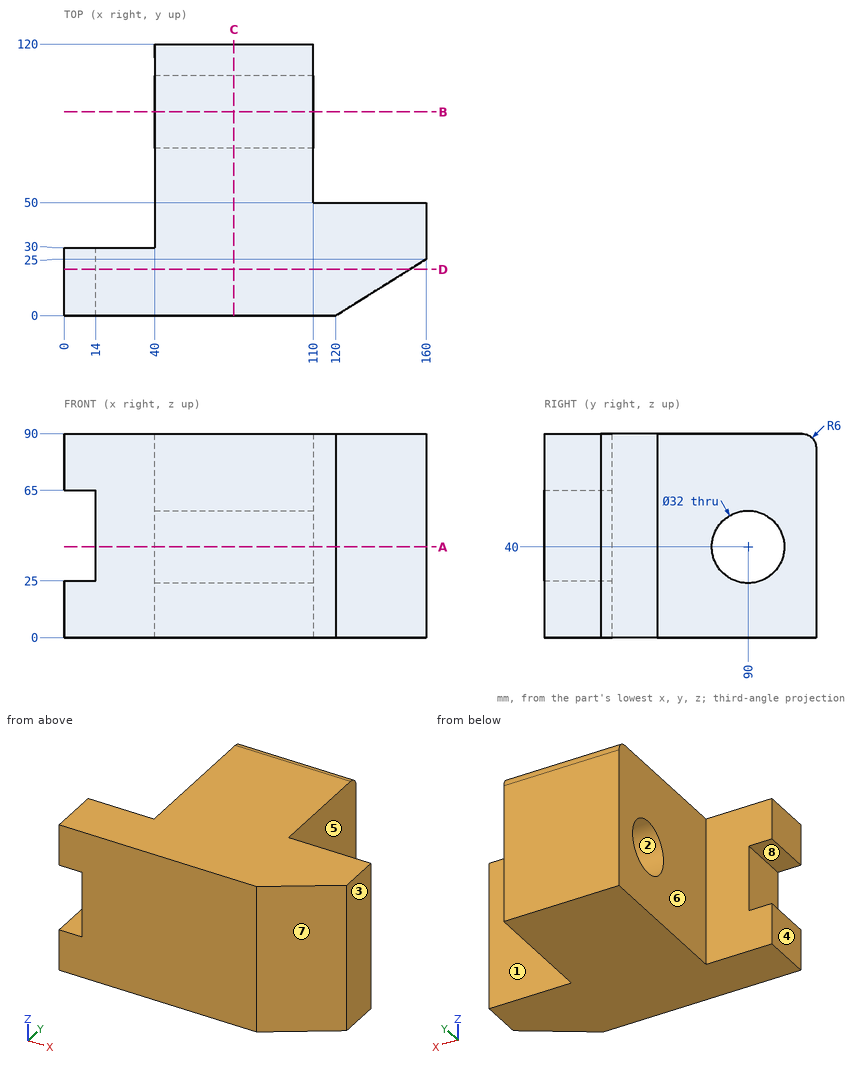
Here's the drawing with two shaded views (mm, measured from the low corner). I have some questions. A direction names the side the tool comes from. Give positions to 0.01 mm unless a question says otherwise; leave off trailing zeros. Loops run counter-clockwise (first coordinate to the right, second up) from the corner with the lowest first, then second, coordinate; pieces in that order, holes last. Notation, with made-up numbers: M 22.25,29 L 42.25,29 A25 ccw 42.25,54 Z; hole C 23.5,-33.75 d1. An arc over 180 degrees is marked long. Use one line per item in the form item = value. Start each with the question number.
(1) I want a section at A-A, the plane z = 40. Write out the boundary of the cut face in (x, y), and give its area (3 significant figures).
(2) I want a section at B-B, the plane y = 90. Write out the boundary of the cut face in (x, z).
(3) Please list where these lines run through material, in increasing order: line 1 (Y direction, x = 79.5, z = 40); line 2 (X direction, y = 77, z = 79.5); line 3 (Y direction, x = 37, z = 72.5).
(4) I'm going to push flat-ended pins straight in: P1, Ø10, axis at y = 46, z = 76, coming from the -X side; P2, Ø20, axis at x = 19.5, z = 54.5, coming from the +Y side; P3, Ø4, axis at x = 48, y = 19.5, coming from the -Z side. Where does each tip first touch, or does it pass through?
(5) Thinking about a two-plate mould opening in Y: for the marked faces 1, 2 and 3, which applies, released by +Y, released by -Y, zero draft, split by the parting line, or undercut?
(6) On a 3-axis mill with a long thin cutter (end or side, diameter ignored), from which of +Z, -Z, +X, -X, +Y, -Y can I reach the whole of each face in a straight line? I mean the marked faces 4, 5, 6, 7 and 8. Say none if no direction works.
(7) I want a section at C-C, the plane x = 75. Write out the boundary of the cut face in (y, z).
(8) I want a section at D-D, the plane y = 20.5. Write out the boundary of the cut face in (x, z).
Worked out:
q1.outline = M 14,0 L 120,0 L 160,25 L 160,50 L 110,50 L 110,74 L 40,74 L 40,30 L 14,30 Z; M 40,106 L 110,106 L 110,120 L 40,120 Z
q1.area = 8,940 mm²
q2.outline = M 40,0 L 110,0 L 110,24 L 40,24 Z; M 40,56 L 110,56 L 110,90 L 40,90 Z
q3.line_1 = 0 to 74, 106 to 120
q3.line_2 = 40 to 110
q3.line_3 = 0 to 30
q4.P1 = 40
q4.P2 = 30
q4.P3 = 0
q5.face_1 = released by +Y
q5.face_2 = undercut
q5.face_3 = zero draft
q6.face_4 = +Z, -Z, -X, +Y, -Y
q6.face_5 = +Z, -Z, +X, +Y
q6.face_6 = +Z, -Z, -X, +Y
q6.face_7 = +Z, -Z, +X, -Y
q6.face_8 = -X, +Y, -Y
q7.outline = M 0,0 L 120,0 L 120,84 A6 ccw 114,90 L 0,90 Z; hole C 90,40 d32
q8.outline = M 0,0 L 152.8,0 L 152.8,90 L 0,90 L 0,65 L 14,65 L 14,25 L 0,25 Z
